```python
from build123d import *

# Parameters (mm, degrees)
F0_W          = 850
F0_H          = 300
F1_DEPTH      = 85
F1_DEPTH_BACK = 85
F2_T          = -1.6
F3_R          = 14
F4_DEPTH      = 20
F5_R          = 7.5
F6_DEPTH      = 10


with BuildPart() as f1:
    # F0 (on Top) → F1 (new body, two sides)
    with BuildSketch(Plane.XY) as f1_sk:
        Rectangle(F0_W, F0_H)
    extrude(amount=F1_DEPTH)
    extrude(f1_sk.sketch, amount=-F1_DEPTH_BACK)

    # F2
    f2_openings = [f1.faces().sort_by_distance(p)[0] for p in [
        (0, 0, 85),
    ]]
    offset(amount=F2_T, openings=f2_openings)

    # F3 (on face) → F4 (join)
    with BuildSketch(Plane.XZ.offset(150)):
        with Locations((400, -69)):
            Circle(F3_R)
    extrude(amount=F4_DEPTH)

    # F5 (on face) → F6 (join)
    with BuildSketch(Plane.XZ.offset(150)):
        with Locations((-410, 55)):
            Circle(F5_R)
    extrude(amount=F6_DEPTH)


solid = f1.part
```
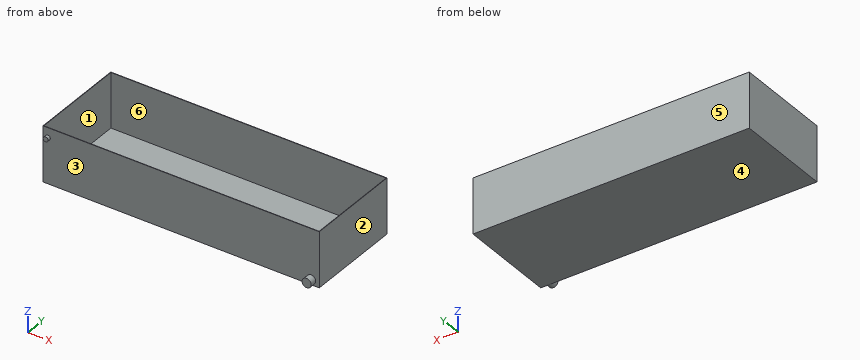
Model file for the job. Use its own axes, mm. Face numbers are marked on the shaded views. A direction names the side the tool comes from. Coordinates: 2 decimals unless noted, no trailing zeros. Order: outer loops, then holes, each group sorted by start corner. A loop starts at its lowest first (then second) coordinate and runs counter-clockwise, first axis right, second up. Notation, with made-up numbers: (44.25, 83.5) -> (82.25, 83.5) arc R20 cw to (82.25, 120.5) -> close; hole circle Ø10 at (-29, -3). An arc over 180 degrees is marked (long way). Answer as a JSON object with one key per item and string values. Group by question number.
1) Which spindle directions (+Z, -Z, +X, -X, +Y, -Y) get a long thin tool onto all of the face, cutting with end or side? Do the marked faces 1 and 2. Say none if no direction does.
2) Cut at C-C, the plane y = 48. Write the cut outline in (x, z).
3) Cut at A-A, the plane z = -4. Write the cut outline in (x, y), then the cut area to 3 significant figures.
4) Cut at B-B, the plane x = 400. Write the cut outline in (y, z), then the cut area to 3 significant figures.
5) Drill centre lines: L1, parallel to X at y = 4, z = 45; L2, parallel to Y at x = -271.5, z = 61; L3, parallel to Z at x = 91.5, y = 130. Where is each one in solid material? Low to high.
6) Flat gauge pins, fed straight in: pin 1 (5 mm diameter, centred on x = -169.5, y = -124, fed in from +Z); pin 2 (7.5 mm diameter, centred on x = -411, z = 52, fed in from -Y); pin 3 (8 mm diameter, centred on x = 136, z = -32.5, fed in from -Y). Where does each tip first touch, or does it go through?
7) Pull direction Y, two halves, no side cores. Call the marked faces 3, 4, 5 and 6: +Y half, -Y half, draft (parallel to the pull), parting line (faces both ways), or undercut.
8) Cut at D-D, the plane z = -69. Write the cut outline in (x, y), then the cut area to 3 significant figures.
Check values:
{
 "1": {"face 1": "+Z", "face 2": "+Z, -Z, +X, +Y, -Y"},
 "2": {"outline": "(-425, -85) -> (425, -85) -> (425, 85) -> (423.4, 85) -> (423.4, -83.4) -> (-423.4, -83.4) -> (-423.4, 85) -> (-425, 85) -> close"},
 "3": {"outline": "(-425, -150) -> (425, -150) -> (425, 150) -> (-425, 150) -> close; hole (-423.4, -148.4) -> (423.4, -148.4) -> (423.4, 148.4) -> (-423.4, 148.4) -> close", "area": "3,670 mm²"},
 "4": {"outline": "(-170, -83) -> (-150, -83) -> (-150, -85) -> (150, -85) -> (150, 85) -> (148.4, 85) -> (148.4, -83.4) -> (-148.4, -83.4) -> (-148.4, 85) -> (-150, 85) -> (-150, -55) -> (-170, -55) -> close", "area": "1,580 mm²"},
 "5": {"L1": "x = -425 to -423.4, 423.4 to 425", "L2": "y = -150 to -148.4, 148.4 to 150", "L3": "z = -85 to -83.4"},
 "6": {"pin 1": "stops at z = -83.4", "pin 2": "stops at y = -160", "pin 3": "stops at y = -150"},
 "7": {"face 3": "-Y half", "face 4": "draft", "face 5": "+Y half", "face 6": "undercut"},
 "8": {"outline": "(-425, -150) -> (386, -150) -> (386, -170) -> (414, -170) -> (414, -150) -> (425, -150) -> (425, 150) -> (-425, 150) -> close; hole (-423.4, -148.4) -> (423.4, -148.4) -> (423.4, 148.4) -> (-423.4, 148.4) -> close", "area": "4,230 mm²"}
}
